Could you check a few things on this model? Use its own coordinates, in mm. Face numbers are marked on the shaded views. A direction names the side the tool comes from. Coordinates: 2 decimals unless noted, no trailing zeros. Write each loop counter-clockwise with the first axis right and the second up, starting at its lowest first coordinate (ties: lowest second). Pieces come first, ordered by that corner, then holes.
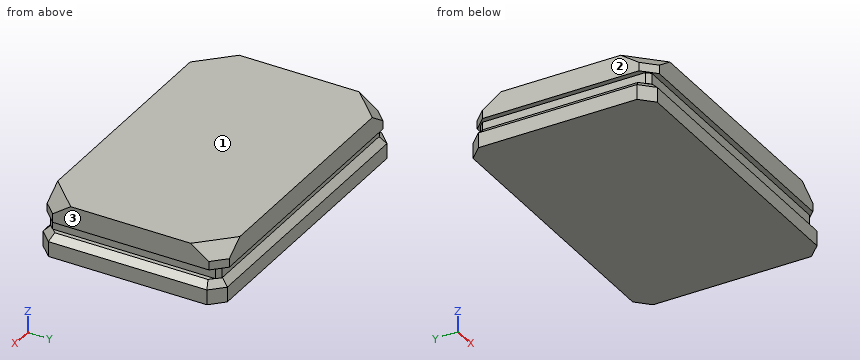
```python
from build123d import *

# Parameters (mm, degrees)
SKETCH_W        = 1400
SKETCH_H        = 860
PAD_DEPTH       = 100
CHAMFER_SIZE    = 60
CHAMFER001_SIZE = 30
SKETCH001_W     = 1300
SKETCH001_H     = 800
PAD001_DEPTH    = 50
CHAMFER002_SIZE = 20
SKETCH002_W     = 1350
SKETCH002_H     = 850
PAD002_DEPTH    = 100
CHAMFER003_SIZE = 60
CHAMFER004_SIZE = 60


with BuildPart() as part:
    # Sketch → Pad (new body)
    with BuildSketch(Plane.XY):
        Rectangle(SKETCH_W, SKETCH_H)
    extrude(amount=PAD_DEPTH)

    # Chamfer
    chamfer_edges = [part.edges().sort_by_distance(p)[0] for p in [
        (-700, 430, 50),
        (700, 430, 50),
        (-700, -430, 50),
        (700, -430, 50),
    ]]
    chamfer(chamfer_edges, length=CHAMFER_SIZE)

    # Chamfer001
    chamfer001_edges = [part.edges().sort_by_distance(p)[0] for p in [
        (-700, 0, 100),
        (-670, 400, 100),
        (0, 430, 100),
        (-670, -400, 100),
        (0, -430, 100),
        (670, -400, 100),
        (700, 0, 100),
        (670, 400, 100),
    ]]
    chamfer(chamfer001_edges, length=CHAMFER001_SIZE)

    # Sketch001 (on Face8 of Chamfer001) → Pad001 (join)
    with BuildSketch(Plane.XY.offset(100)):
        Rectangle(SKETCH001_W, SKETCH001_H)
    extrude(amount=PAD001_DEPTH)

    # Chamfer002
    chamfer002_edges = [part.edges().sort_by_distance(p)[0] for p in [
        (650, 400, 125),
        (650, -400, 125),
        (-650, 400, 125),
        (-650, -400, 125),
    ]]
    chamfer(chamfer002_edges, length=CHAMFER002_SIZE)

    # Sketch002 (on Face5 of Chamfer002) → Pad002 (join)
    with BuildSketch(Plane.XY.offset(150)):
        Rectangle(SKETCH002_W, SKETCH002_H)
    extrude(amount=PAD002_DEPTH)

    # Chamfer003
    chamfer003_edges = [part.edges().sort_by_distance(p)[0] for p in [
        (675, 425, 200),
        (-675, 425, 200),
        (-675, -425, 200),
        (675, -425, 200),
    ]]
    chamfer(chamfer003_edges, length=CHAMFER003_SIZE)

    # Chamfer004
    chamfer004_edges = [part.edges().sort_by_distance(p)[0] for p in [
        (645, 395, 250),
        (645, -395, 250),
        (-645, -395, 250),
        (-645, 395, 250),
    ]]
    chamfer(chamfer004_edges, length=CHAMFER004_SIZE)


solid = part.part
```
1. On a 3-axis mill with a long thin cutter (end or side, diameter ignored), from which of +Z, -Z, +X, -X, +Y, -Y can I reach the whole of each face in a straight line? I mean the marked faces 1, 2 and 3. Say none if no direction works.
Verdict:
face 1: +Z, +X, -X, +Y, -Y
face 2: +Z, -X, +Y, -Y
face 3: +Z, +X, +Y, -Y
2. I want a section at D-D on z = 235. Please give me the cut outline in (x, y), plus the area to 3 significant figures.
Verdict:
outline: (-675, -301.36) - (-551.36, -425) - (551.36, -425) - (675, -301.36) - (675, 301.36) - (551.36, 425) - (-551.36, 425) - (-675, 301.36) - close
area: 1,120,000 mm2
3. I want a section at B-B on y = -144.5. Please give me the cut outline in (x, z), plus the area to 3 significant figures.
Verdict:
outline: (-700, 0) - (700, 0) - (700, 70) - (670, 100) - (650, 100) - (650, 150) - (675, 150) - (675, 250) - (-675, 250) - (-675, 150) - (-650, 150) - (-650, 100) - (-670, 100) - (-700, 70) - close
area: 339,000 mm2
4. For pin 1 (1 mm diameter, centred on y = -53.5, z = 75, fed in from +X); pin 2 (5 mm diameter, centred on y = 288, z = 74, fed in from +X); pin 3 (4 mm diameter, centred on x = 112, z = 133, fed in from +Y), each with a flat end and sliding along its axis, tell me the tip position at first contact or that it passes through.
Verdict:
pin 1: stops at x = 695.5
pin 2: stops at x = 698.5
pin 3: stops at y = 400
5. Please list where these lines run through material, in increasing order: line 1 along X through (y, z) = (-34, 156.5); line 2 along Y through (x, z) = (101, 187); line 3 along X through (y, z) = (333, 119.5).
Verdict:
line 1: x = -675 to 675
line 2: y = -425 to 425
line 3: x = -650 to 650
6. I want a section at A-A on z = 171. Please give me the cut outline in (x, y).
Verdict:
outline: (-675, -365) - (-615, -425) - (615, -425) - (675, -365) - (675, 365) - (615, 425) - (-615, 425) - (-675, 365) - close
7. I want a section at C-C on x = -437.5. Please give me the cut outline in (y, z), plus the area to 3 significant figures.
Verdict:
outline: (-430, 0) - (430, 0) - (430, 70) - (400, 100) - (400, 150) - (425, 150) - (425, 250) - (-425, 250) - (-425, 150) - (-400, 150) - (-400, 100) - (-430, 70) - close
area: 210,000 mm2
